```python
from build123d import *

# Parameters (mm, degrees)
ESBO_O1_W                = 60
ESBO_O1_H                = 20
RESSALTO_EXTRUS_O1_DEPTH = 40
ESBO_O2_W                = 20
ESBO_O2_H                = 20
CORTE_EXTRUS_O1_DEPTH    = 40
ESBO_O3_W                = 60
ESBO_O3_H                = 40.21646748
RESSALTO_EXTRUS_O2_DEPTH = 30
ESBO_O4_W                = 20
ESBO_O4_H                = 30
CORTE_EXTRUS_O4_DEPTH    = 20
ESBO_O7_W                = 20
ESBO_O7_H                = 30
CORTE_EXTRUS_O6_DEPTH    = 10


with BuildPart() as part:
    # Esboço1 → Ressalto-extrusão1 (new body)
    with BuildSketch(Plane.XY):
        with Locations((30, 10)):
            Rectangle(ESBO_O1_W, ESBO_O1_H)
    extrude(amount=RESSALTO_EXTRUS_O1_DEPTH)

    # Esboço2 → Corte-extrusão1 (cut)
    with BuildSketch(Plane(origin=(0, 20, 0), x_dir=(1, 0, 0), z_dir=(0, 1, 0))):
        with Locations((30, -30)):
            Rectangle(ESBO_O2_W, ESBO_O2_H)
    extrude(amount=-CORTE_EXTRUS_O1_DEPTH, mode=Mode.SUBTRACT)

    # Esboço3 → Ressalto-extrusão2 (add)
    with BuildSketch(Plane(origin=(0, 0, 0), x_dir=(-1, 0, 0), z_dir=(0, 0, -1))):
        with Locations((-30, 20.10823374)):
            Rectangle(ESBO_O3_W, ESBO_O3_H)
    extrude(amount=RESSALTO_EXTRUS_O2_DEPTH)

    # Esboço4 → Corte-extrusão4 (cut)
    with BuildSketch(Plane(origin=(0, 40.21646748, 0), x_dir=(1, 0, 0), z_dir=(0, 1, 0))):
        with Locations((30, 15)):
            Rectangle(ESBO_O4_W, ESBO_O4_H)
    extrude(amount=-CORTE_EXTRUS_O4_DEPTH, mode=Mode.SUBTRACT)

    # Esboço7 → Corte-extrusão6 (cut)
    with BuildSketch(Plane(origin=(0, 40.21646748, 0), x_dir=(1, 0, 0), z_dir=(0, 1, 0))):
        with Locations((50, 15)):
            Rectangle(ESBO_O7_W, ESBO_O7_H)
    extrude(amount=-CORTE_EXTRUS_O6_DEPTH, mode=Mode.SUBTRACT)


solid = part.part
```
Design review of the part built by this model. Coordinates are the model's own, in mm. A direction names the side the tool comes from. Give positions to 0.01 mm unless a question says otherwise; leave off trailing zeros. Loops run counter-clockwise (first coordinate to the right, second up) from the corner with the lowest first, then second, coordinate; pieces in that order, holes last. Notation, with made-up numbers: M 15,-30.5 L 60,-30.5 A17 cw 60,-8.5 Z; hole C 29,-6.75 d9. An arc over 180 degrees is marked long. Return JSON: item names as keys, results as strings. Group by question number.
Item 1: Insertion check: pin 1 Ø2 at (x, z) = (49, 22.5) entering from +Y; pin 2 Ø22 at (x, z) = (49.5, -8) entering from +Y; pin 3 Ø6 at (x, z) = (30, -20.5) entering from +Y. Each pin has a flat end and moves straight along its axis. Give the tip position at first contact, or say it passes through.
Item 2: We need section C-C (x = 10). Give the boundary of the cut face in (y, z), and give its area (3 significant figures).
Item 3: For probe 1 along X at (y, z) = (23.5, -4.5); probe 2 along Y at (x, z) = (13.5, 32), list the stretches that pass through material, from the lowest coordinate up.
Item 4: Tool access review of faces 1 (the flat face through (50, 30.216, -15)), 2 (the flat face through (29.6, 20, 19.7)), 3 (the flat face through (40, 10, 30)), 4 (the flat face through (30, 20.216, -15)): name each direction out of +Z, -Z, +X, -X, +Y, -Y from which nothing blocks a thin tool from reaching the whole face with its end or side.
Item 5: We need section B-B (z = -14). Give the boundary of the cut face in (x, y), and give its area (3 significant figures).
Item 6: We need section A-A (y = 22). Give the boundary of the cut face in (x, z), and give its area (3 significant figures).
Item 7: Mouldability with a two-part tool opening along X and no side actions: class faces 5 (the flat face through (20, 10, 30)), 6 (the flat face through (50, 10, 40)), 7 (the flat face through (60, 12, 5)), 8 (the flat face through (0, 15, -2)) as released by +X, released by -X, zero draft, split by the parting line, or undercut.
Item 8: We need section D-D (y = 10.5). Give the boundary of the cut face in (x, z).
Output:
{
 "1": {"pin 1": "stops at y = 20", "pin 2": "stops at y = 30.22", "pin 3": "stops at y = 20.22"},
 "2": {"outline": "M 0,-30 L 40.22,-30 L 40.22,0 L 20,0 L 20,40 L 0,40 Z", "area": "2,010 mm^2"},
 "3": {"probe 1": "x = 0 to 20, 40 to 60", "probe 2": "y = 0 to 20"},
 "4": {"face 1": "+Z, -Z, +X, +Y", "face 2": "+Z, +X, -X, +Y", "face 3": "+Z, +Y, -Y", "face 4": "+Z, -Z, +Y"},
 "5": {"outline": "M 0,0 L 60,0 L 60,30.22 L 40,30.22 L 40,20.22 L 20,20.22 L 20,40.22 L 0,40.22 Z", "area": "1,810 mm^2"},
 "6": {"outline": "M 0,-30 L 20,-30 L 20,0 L 0,0 Z; M 40,-30 L 60,-30 L 60,0 L 40,0 Z", "area": "1,200 mm^2"},
 "7": {"face 5": "undercut", "face 6": "zero draft", "face 7": "released by +X", "face 8": "released by -X"},
 "8": {"outline": "M 0,-30 L 60,-30 L 60,40 L 40,40 L 40,20 L 20,20 L 20,40 L 0,40 Z"}
}
